Geometry check sheet. Reference: drawing and pictorial views, mm from the part's lowest x, y, z. A direction names the side the tool comes from. Give positions to 0.01 mm unless a question says otherwise; leave off trailing zeros. Write each loop counter-clockwise with the first axis right and the second up, starting at its lowest first coordinate (ties: lowest second). Pieces come first, ordered by that corner, then holes. Notation, with made-up numbers: M 21,1.25 L 65,1.25 A19 ccw 65,18.25 Z; hole C 83.5,85.5 d7. An arc over 180 degrees is marked long. Answer as a JSON object with one key per item and string values.
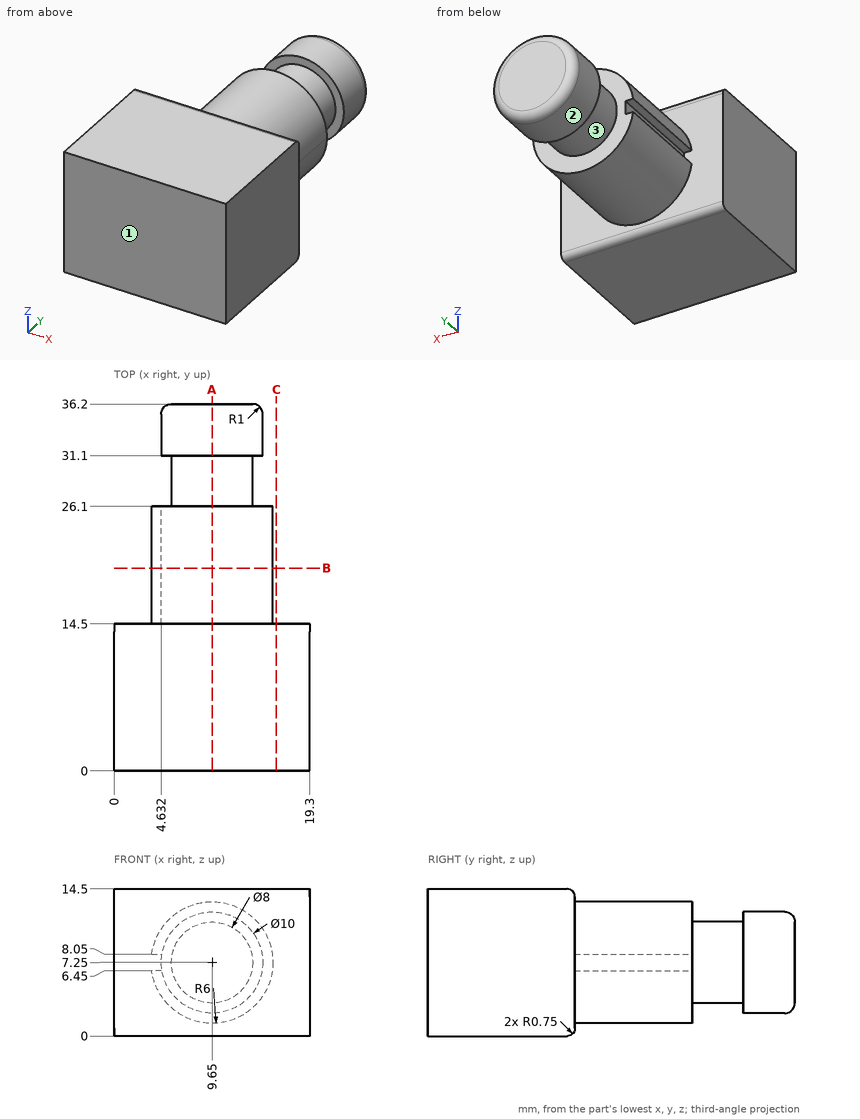
1) Go/stop test with flat-tipped pins: pin 1 (5 mm diameter, centred on x = 14.5, z = 10, fed in from +Y); pin 2 (1.5 mm diameter, centred on y = 24, z = 12, fed in from -X); pin 3 (6 mm diameter, centred on x = 10, y = 21, fed in from -Z); pin 4 (0.5 mm diameter, centred on x = 4, y = 21, fed in from -Z) (1 decimal). Record where each tip stops, or that it passes through.
Completed:
{"pin 1": "stops at y = 36.2", "pin 2": "stops at x = 5.18", "pin 3": "stops at z = 1.25", "pin 4": "stops at z = 4.6"}
2) Section check C-C on x = 16. Record the boundary of the cut face in (y, z), and give its area (3 significant figures).
Completed:
{"outline": "M 0,0 L 13.75,0 A0.75 ccw 14.5,0.75 L 14.5,13.75 A0.75 ccw 13.75,14.5 L 0,14.5 Z", "area": "210 mm2"}
3) Section check B-B on y = 20. Record the boundary of the cut face in (x, z), and give its area (3 significant figures).
Completed:
{"outline": "M 3.7,6.45 A6 ccw long 3.7,8.05 L 4.63,8.05 L 4.63,6.45 Z", "area": "112 mm2"}
4) Thickness scan on L1, parallel to Y at x = 5, z = 7.5 (1 decimal); L2, parallel to Y at x = 8.25, z = 13.5; L3, parallel to X at y = 28, z = 7. Record the ranges inside material, lowest first.
Completed:
{"L1": "y = 0 to 26.1, 31.1 to 36", "L2": "y = 0 to 14.5", "L3": "x = 5.66 to 13.64"}
5) Section check A-A on x = 9.65. Record the boundary of the cut face in (y, z).
Completed:
{"outline": "M 0,0 L 13.75,0 A0.75 ccw 14.5,0.75 L 14.5,1.25 L 26.1,1.25 L 26.1,3.25 L 31.1,3.25 L 31.1,2.25 L 35.2,2.25 A1 ccw 36.2,3.25 L 36.2,11.25 A1 ccw 35.2,12.25 L 31.1,12.25 L 31.1,11.25 L 26.1,11.25 L 26.1,13.25 L 14.5,13.25 L 14.5,13.75 A0.75 ccw 13.75,14.5 L 0,14.5 Z"}
6) Access from +Z, -Z, +X, -X, +Y, -Y to the whole of each face (thin tool, end or side, straight path). Record for the marked faces 1, 2 and 3.
Completed:
{"face 1": "+Z, -Z, +X, -X, -Y", "face 2": "+Y", "face 3": "none"}
